Read the model definition and answer for the solid it produces. Units are mm, in the model's axes. Face numbers are marked on the shaded views. A direction names the side the tool comes from. Coordinates: 2 decimals unless noted, no trailing zeros. Write each loop counter-clockwise with the first axis right and the second up, starting at its lowest first coordinate (ties: lowest second). Pieces come first, ordered by that corner, then holes.
(1) Section B-B on z = 30 is taken. Write down the section's boundary in (x, y).
(2) Section C-C on y = 27.5 is taken. Write down the section's boundary in (x, z) (3 decimals).
(3) Find the intervals of material crossed by probe 1 along Z at (x, y) = (3.75, 42); probe 2 along Y at (x, z) = (-4, -44); probe 3 along X at (y, z) = (-6, 37), in increasing order.
(4) Section A-A on x = 1.25 is taken. Write down the section's boundary in (y, z) (3 decimals).
(5) Section D-D on y = -8.5 is taken. Write down the section's boundary in (x, z), then the cut area to 3 significant figures.
(6) Which of the six approach directions +Z, -Z, +X, -X, +Y, -Y give full straight-line access (tool end or side, diameter ignored) to the marked faces 1, 2 and 3?
(7) Given pin 1 (5 mm diameter, centred on x = -1, z = 57, fed in from -Y); pin 2 (1.9 mm diameter, centred on y = 38, z = -58, fed in from -X); pin 3 (1.6 mm diameter, centred on x = -4, y = 33.5, fed in from -Z), each flat-ended and moving along its own axis, determine where each tip first touches the part or whether it passes through.
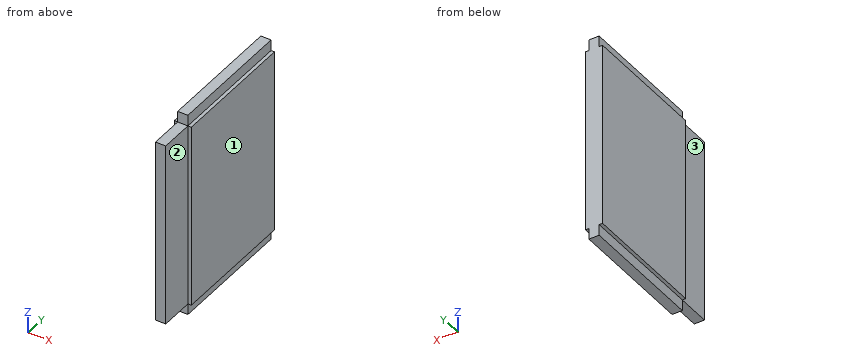
Autodesk Inventor part; units mm, degrees
ref_plane "YZ Plane" through (0, 0, 0) normal (1, 0, 0) x (0, 1, 0)
ref_plane "XZ Plane" through (0, 0, 0) normal (0, 1, 0) x (-1, 0, 0)
ref_plane "XY Plane" through (0, 0, 0) normal (0, 0, 1) x (1, 0, 0)
sketch "Sketch1" plane through (0, 0, 0) normal (0, 1, 0) x (-1, 0, 0)
  point P0 (0, 0)
sketch "Sketch2" plane through (0, 0, 0) normal (0, 1, 0) x (-1, 0, 0)
  line L0 (5, 54.202) -> (-5, 54.202)
  line L1 (-5, 54.202) -> (-5, -54.202)
  line L2 (-5, -54.202) -> (5, -54.202)
  line L3 (5, -54.202) -> (5, 54.202)
  line L4 (5, 54.202) -> (-5, -54.202) construction
  line L5 (-5, 54.202) -> (5, -54.202) construction
  line L6 (3, 60.655) -> (-3, 60.655)
  line L7 (-3, 60.655) -> (-3, -60.655)
  line L8 (-3, -60.655) -> (3, -60.655)
  line L9 (3, -60.655) -> (3, 60.655)
  line L10 (3, 60.655) -> (-3, -60.655) construction
  line L11 (-3, 60.655) -> (3, -60.655) construction
  point P0 (0, 0)
  point P1 (3, 54.202)
  point P2 (-3, 54.202)
  point P3 (-3, -54.202)
  point P4 (3, -54.202)
  dimension "d0" = 10
  dimension "d1" = 108.404
  dimension "d2" = 6
  dimension "d3" = 121.31
extrude "Extrusion1" add sketch "Sketch2" along normal blind 75
extrude "Extrusion2" add sketch "Sketch2" against normal blind 20 contours L9 L2 L7 L0
properties part number "sciana_bezdziury" material "ABS Plastic"
Response:
1. outline: (-5, 0) - (-3, 0) - (-3, -20) - (3, -20) - (3, 0) - (5, 0) - (5, 75) - (-5, 75) - close
2. outline: (-5, -54.202) - (-3, -54.202) - (-3, -60.655) - (3, -60.655) - (3, -54.202) - (5, -54.202) - (5, 54.202) - (3, 54.202) - (3, 60.655) - (-3, 60.655) - (-3, 54.202) - (-5, 54.202) - close
3. probe 1: z = -54.2 to 54.2
3. probe 2: y = 0 to 75
3. probe 3: x = -3 to 3
4. outline: (-20, -54.202) - (0, -54.202) - (0, -60.655) - (75, -60.655) - (75, 60.655) - (0, 60.655) - (0, 54.202) - (-20, 54.202) - close
5. outline: (-3, -54.2) - (3, -54.2) - (3, 54.2) - (-3, 54.2) - close
5. area: 650 mm2
6. face 1: +Z, -Z, +X, +Y, -Y
6. face 2: +Z, -Z, +X, -Y
6. face 3: +Z, -Z, -X, -Y
7. pin 1: stops at y = 0
7. pin 2: stops at x = -3
7. pin 3: stops at z = -54.2
